Geometry check sheet. Reference: drawing and pictorial views, mm from the part's lowest x, y, z. A direction names the side the tool comes from. Coordinates: 2 decimals unless noted, no trailing zeros. Write each loop counter-clockwise with the first axis right and the second up, starting at its lowest first coordinate (ties: lowest second). Pieces come first, ordered by that corner, then holes. Notation, with made-up numbers: (53.25, 68) -> (66.25, 68) arc R19 cw to (66.25, 92) -> close; hole circle Ø4 at (54, 62). An arc over 180 degrees is marked (long way). Put each result on its own line as item: value.
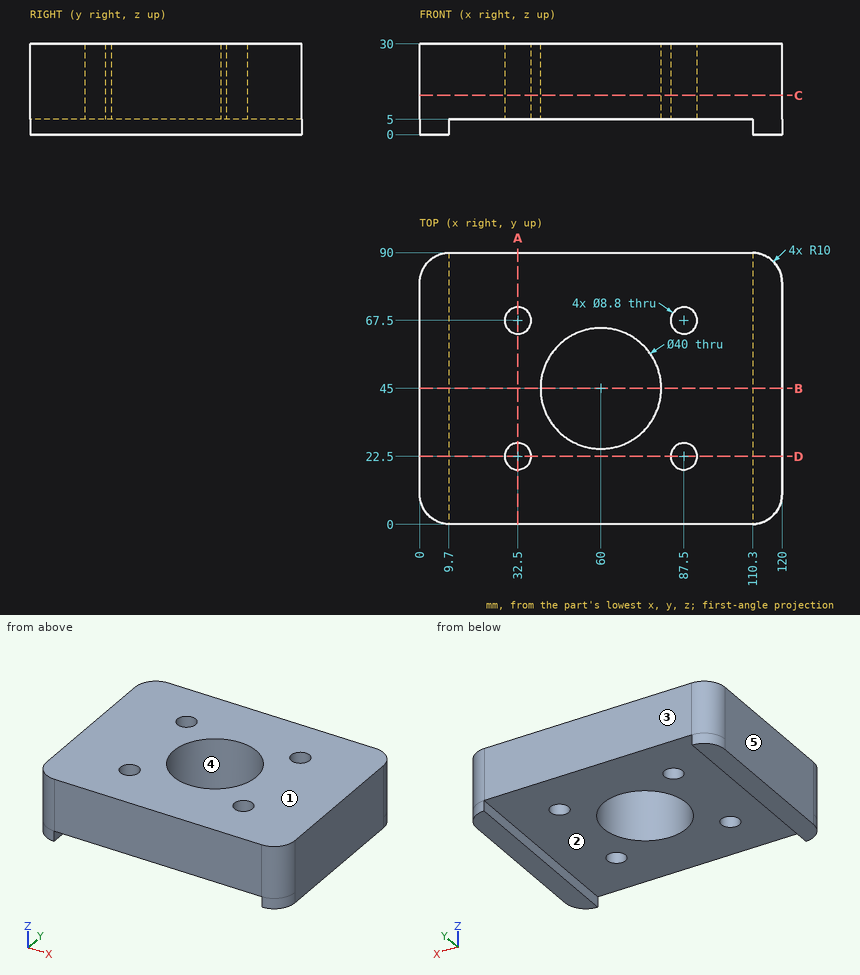
Q1. Depth check by flat-ended pin: P1, Ø2, axis at x = 98.5, y = 64.5, coming from the -Z side. Enter the tip coordinate at first touch or a pass-through.
Recorded:
P1: stops at z = 5
Q2. Cross-section at C-C (z = 13). Record the cut outline in (x, y), plus the area to 3 significant figures.
Recorded:
outline: (0, 10) arc R10 ccw to (10, 0) -> (110, 0) arc R10 ccw to (120, 10) -> (120, 80) arc R10 ccw to (110, 90) -> (10, 90) arc R10 ccw to (0, 80) -> close; hole circle Ø8.8 at (32.5, 22.5); hole circle Ø8.8 at (32.5, 67.5); hole circle Ø40 at (60, 45); hole circle Ø8.8 at (87.5, 22.5); hole circle Ø8.8 at (87.5, 67.5)
area: 9,210 mm2
Q3. Mould release check, pull along X, two halves, no side actions. Record for the marked faces 3, 4 and 5: released by +X, released by -X, zero draft, split by the parting line, or undercut.
Recorded:
face 3: zero draft
face 4: undercut
face 5: released by -X
Q4. Cross-section at B-B (y = 45). Record the cut outline in (x, z), plus the area to 3 significant figures.
Recorded:
outline: (0, 0) -> (9.7, 0) -> (9.7, 5) -> (40, 5) -> (40, 30) -> (0, 30) -> close; (80, 5) -> (110.3, 5) -> (110.3, 0) -> (120, 0) -> (120, 30) -> (80, 30) -> close
area: 2,100 mm2
Q5. Tool access check on the marked faces 1 and 2. Record the directions out of +Z, -Z, +X, -X, +Y, -Y that give a thin tool (end or side, any length) a straight path to the whole face; none if there is none.
Recorded:
face 1: +Z, +X, -X, +Y, -Y
face 2: -Z, +Y, -Y
Q6. Cross-section at D-D (y = 22.5). Record the cut outline in (x, z).
Recorded:
outline: (0, 0) -> (9.7, 0) -> (9.7, 5) -> (28.1, 5) -> (28.1, 30) -> (0, 30) -> close; (36.9, 5) -> (83.1, 5) -> (83.1, 30) -> (36.9, 30) -> close; (91.9, 5) -> (110.3, 5) -> (110.3, 0) -> (120, 0) -> (120, 30) -> (91.9, 30) -> close
Q7. Material ranges on line 1 along Y through (x, z) = (32.5, 23.75); line 2 along X through (y, z) = (67, 10.5); line 3 along X through (y, z) = (21.5, 13.75), recorded low to high.
Recorded:
line 1: y = 0 to 18.1, 26.9 to 63.1, 71.9 to 90
line 2: x = 0 to 28.13, 36.87 to 83.13, 91.87 to 120
line 3: x = 0 to 28.22, 36.78 to 83.22, 91.78 to 120
Q8. Cross-section at A-A (x = 32.5). Record the cut outline in (y, z).
Recorded:
outline: (0, 5) -> (18.1, 5) -> (18.1, 30) -> (0, 30) -> close; (26.9, 5) -> (63.1, 5) -> (63.1, 30) -> (26.9, 30) -> close; (71.9, 5) -> (90, 5) -> (90, 30) -> (71.9, 30) -> close
